Input: part model. Units: mm. Frame: model coordinates. A direction names the side the tool comes from. Coordinates: 2 decimals unless noted, no trailing zeros. Order: outer loops, then holes, each group sorted by start corner. A loop starts at its lowest first (then second) coordinate and runs counter-clockwise, first axis right, second up. Notation, with made-up numbers: (39.25, -20) -> (46.25, -20) arc R31 cw to (46.25, 18) -> close; hole circle Ø10 at (5, 76.5). An arc over 180 degrees is marked (long way). Answer as CSV lines item,"result".
from build123d import *

# Parameters (mm, degrees)
F1_DEPTH    = 5
F2_W        = 9.5
F2_H        = 1.5
F3_DEPTH    = 12
F4_T1_DEPTH = 14.6433659759


# Not quite as in the source:
# - a fillet or chamfer that OpenCascade refuses, or shapes differently, is made with other operations: its cross-section is extruded or revolved along the edge and cut away or added


with BuildPart() as f1:
    # F0 (on Top) → F1 (new body)
    with BuildSketch(Plane.XY):
        Polygon((-2.5628354418, 5), (-27.6419919184, 5), (-27.6419919184, -5), (-2.5628354418, -5), (-2.5628354418, -10), (7.4371645582, 0), (-2.5628354418, 10), align=None)
    extrude(amount=F1_DEPTH)

    # F2 (on face) → F3 (join)
    with BuildSketch(Plane(origin=(0, 0, 0), x_dir=(1, 0, 0), z_dir=(0, 0, -1))):
        with Locations((-15.3186318129, -0.1973686223)):
            Rectangle(F2_W, F2_H)
    extrude(amount=F3_DEPTH)

    # F4: chamfer of 1 on 2 edges, made by hand

    # F4_s2 → F4_t1 (cut)
    with BuildSketch(Plane.YZ.offset(-22.6403148009)):
        Polygon((0.9473686223, -11), (-0.0526313777, -12), (0.9473686223, -12), align=None)
        Polygon((-0.5526313777, -11), (0.4473686223, -12), (-0.5526313777, -12), align=None)
    extrude(amount=F4_T1_DEPTH, mode=Mode.SUBTRACT)


solid = f1.part
1. Cut plane D-D (x = -7.5). Return the cut outline in (y, z).
Findings:
outline,"(-5, 0) -> (5, 0) -> (5, 5) -> (-5, 5) -> close"
2. Ray query, line 1 along Z through (x, y) = (-23.5, -2.25); line 2 along Y through (x, z) = (-8, 4); line 3 along Y through (x, z) = (-16, -9.75). Return the intervals inside material, ascending.
Findings:
line 1,"z = 0 to 5"
line 2,"y = -5 to 5"
line 3,"y = -0.55 to 0.95"
3. Cut plane C-C (y = 2.25). Return the cut outline in (x, z).
Findings:
outline,"(-27.64, 0) -> (5.19, 0) -> (5.19, 5) -> (-27.64, 5) -> close"
4. Cut plane B-B (z = 0.75). Return the cut outline in (x, y), plus the area to 3 significant figures.
Findings:
outline,"(-27.64, -5) -> (-2.56, -5) -> (-2.56, -10) -> (7.44, 0) -> (-2.56, 10) -> (-2.56, 5) -> (-27.64, 5) -> close"
area,"351 mm2"
5. Contact query for flat-ended pins moving along their axis: pin 1 (1.5 mm diameter, centred on x = -23, y = -4.5, fed in from -Z); pin 2 (1.5 mm diameter, centred on y = 4.5, z = -0.5, fed in from +X); pin 3 (4 mm diameter, centred on x = -13, z = 3.5, fed in from -Y). Output: stop coordinate, or through.
Findings:
pin 1,"stops at z = 0"
pin 2,"stops at x = 3.5"
pin 3,"stops at y = -5"
6. Reachability of faces 1 (the face through (-10.569, 0, -6)), 2 (the face through (-15, 0.947, -5)), 3 (the face through (-20.069, 0, -6)), 4 (the face through (-15, -5, 2)) from +Z, -Z, +X, -X, +Y, -Y: full face, straight path, thin tool, end or side. Return the list, or none.
Findings:
face 1,"-Z, +X, +Y, -Y"
face 2,"-Z, +X, -X, +Y"
face 3,"-Z, -X, +Y, -Y"
face 4,"+Z, -Z, -X, -Y"
7. Cut plane A-A (x = -15.5). Return the cut outline in (y, z).
Findings:
outline,"(-5, 0) -> (-0.55, 0) -> (-0.55, -11) -> (0.2, -11.75) -> (0.95, -11) -> (0.95, 0) -> (5, 0) -> (5, 5) -> (-5, 5) -> close"
